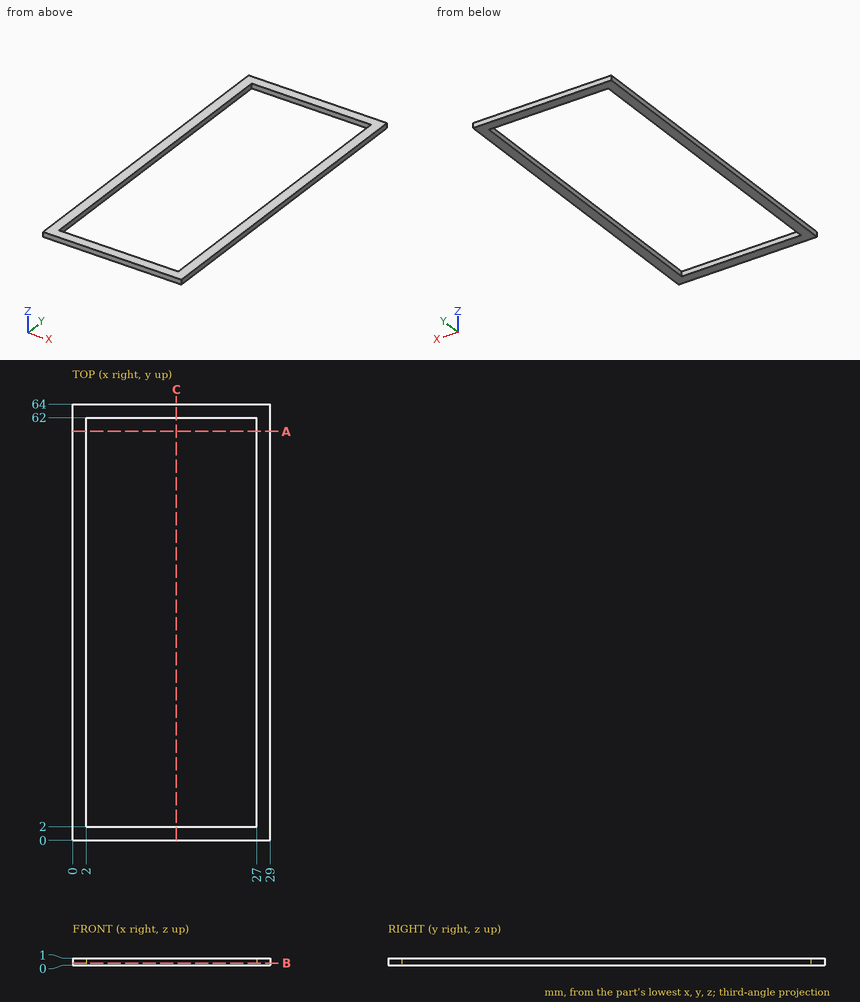
Can you work these out from the drawing? Everything is in mm from the part's minimum corner. Give positions to 0.01 mm unless a question says otherwise; leave off trailing zeros. Order: outer loops, then holes, each group sorted by start corner. A loop starts at its lowest first (then second) coordinate and runs counter-clockwise, first axis right, second up. Notation, with made-up numbers: M 63.25,-4 L 108.25,-4 A34 ccw 108.25,33 Z; hole C 65,52.5 d8. An arc over 180 degrees is marked long. Write item = value, one per line. Start each with the question number.
Q1. Suppose I cut it at C-C (x = 15.25). Write out the boundary of the cut face in (y, z).
Q2. Suppose I cut it at A-A (y = 60). Write out the boundary of the cut face in (x, z), plus the area to 3 significant figures.
Q3. Will these pins go through, and if not, where does the flat tip stop? pin 1 Ø4 at (x, y) = (24, 50) entering from -Z; pin 2 Ø12 at (x, y) = (7.5, 55) entering from -Z.
Q4. I need wall thicknesses on probe 1 along X at (y, z) = (43, 0.35); probe 2 along Y at (x, z) = (8.5, 0.3). Which ranges of each line are inside material? Lowest first, please. Write a range as [from, to].
Q5. Suppose I cut it at B-B (z = 0.3). Write out the boundary of the cut face in (x, y), plus the area to 3 significant figures.
Check result:
q1.outline = M 0,0 L 2,0 L 2,1 L 0,1 Z; M 62,0 L 64,0 L 64,1 L 62,1 Z
q2.outline = M 0,0 L 2,0 L 2,1 L 0,1 Z; M 27,0 L 29,0 L 29,1 L 27,1 Z
q2.area = 4.00 mm2
q3.pin_1 = through
q3.pin_2 = 0
q4.probe_1 = [0, 2], [27, 29]
q4.probe_2 = [0, 2], [62, 64]
q5.outline = M 0,0 L 29,0 L 29,64 L 0,64 Z; hole M 2,2 L 27,2 L 27,62 L 2,62 Z
q5.area = 356 mm2
